from build123d import *

# Parameters (mm, degrees)
SKETCH1_W           = 135
SKETCH1_H           = 122
BOSS_EXTRUDE1_DEPTH = 5.7
CUT_EXTRUDE1_DEPTH  = 57


with BuildPart() as part:
    # Sketch1 → Boss-Extrude1 (new body)
    with BuildSketch(Plane(origin=(0, 0, 0), x_dir=(0, 0, -1), z_dir=(1, 0, 0))):
        with Locations((67.5, 61)):
            Rectangle(SKETCH1_W, SKETCH1_H)
    extrude(amount=BOSS_EXTRUDE1_DEPTH)

    # Sketch2 → Cut-Extrude1 (cut)
    with BuildSketch(Plane(origin=(0, 0, 0), x_dir=(0, 0, -1), z_dir=(1, 0, 0))):
        Polygon((0, 116), (26.9, 116), (26.9, 121.8), (54.1, 121.8), (54.1, 116), (80.9, 116), (80.9, 121.8), (108.1, 121.8), (108.1, 116), (135, 116), (135, 130), (0, 130), align=None)
        Polygon((0, -8), (0, 6), (26.9, 6), (26.9, 0.2), (54.1, 0.2), (54.1, 6), (80.9, 6), (80.9, 0.2), (108.1, 0.2), (108.1, 6), (135, 6), (135, -8), align=None)
    extrude(amount=CUT_EXTRUDE1_DEPTH, mode=Mode.SUBTRACT)


solid = part.part
CAD build for the part. Positions are in the model's coordinates, mm. A direction names the side the tool comes from. Coordinates: 2 decimals unless noted, no trailing zeros. Order: outer loops, then holes, each group sorted by start corner. A loop starts at its lowest first (then second) coordinate and runs counter-clockwise, first axis right, second up.
Item 1: Pin check, flat tips, straight feed: pin 1 Ø3 at (x, z) = (2, -120.5) entering from -Y; pin 2 Ø3 at (x, y) = (3.5, 118) entering from -Z; pin 3 Ø3 at (x, z) = (2.5, -123) entering from +Y. Stop position of each tip, or through.
Check sheet entries:
pin 1: stops at y = 6
pin 2: stops at z = -108.1
pin 3: stops at y = 116
Item 2: Band-saw the part on A-A on x = 4.45. List the corners of the cut face in (y, z).
Check sheet entries:
outline: (0.2, -108.1) - (6, -108.1) - (6, -135) - (116, -135) - (116, -108.1) - (121.8, -108.1) - (121.8, -80.9) - (116, -80.9) - (116, -54.1) - (121.8, -54.1) - (121.8, -26.9) - (116, -26.9) - (116, 0) - (6, 0) - (6, -26.9) - (0.2, -26.9) - (0.2, -54.1) - (6, -54.1) - (6, -80.9) - (0.2, -80.9) - close
Item 3: Two-plate mould, pull along Z, no slides. Class faces 4 (the face through (3, 116, -67)), 5 (the face through (3, 0.2, -40)), 6 (the face through (3, 119, -108.1)): +Z half, -Z half, draft (parallel to the pull), parting line (faces both ways), or undercut.
Check sheet entries:
face 4: undercut
face 5: draft
face 6: -Z half
Item 4: Band-saw the part on B-B on z = -10.5. List the corners of the cut face in (x, y).
Check sheet entries:
outline: (0, 6) - (5.7, 6) - (5.7, 116) - (0, 116) - close
Item 5: 3-axis set-ups, long thin cutter, end or side, ignore diameter. For faces 1 (the face through (3, 3, -80.9)), 2 (the face through (3, 6, -121)), 3 (the face through (3, 3, -26.9)): which of +Z, -Z, +X, -X, +Y, -Y reach the whole face in a straight line?
Check sheet entries:
face 1: +X, -X, -Y
face 2: -Z, +X, -X, -Y
face 3: +Z, +X, -X, -Y
Item 6: Drill centre lines: L1, parallel to Y at x = 5.35, z = -21; L2, parallel to Z at x = 3.1, y = 117.5. Where is each one in solid material? Low to high.
Check sheet entries:
L1: y = 6 to 116
L2: z = -108.1 to -80.9, -54.1 to -26.9
